from build123d import *

# Parameters (mm, degrees)
F1_DEPTH         = 1
F4_DEPTH         = 0.7
F4_COPIES2_COUNT = 2
F5_W             = 38
F5_H             = 12
F6_DEPTH         = 3
F7_R             = 1.5


# Not quite as in the source:
# - a pattern or mirror of a feature is missing from the dataset's text; its kind, count and spacing are read off the source's solid


with BuildPart() as f1:
    # F0 (on Front) → F1 (new body, symmetric)
    with BuildSketch(Plane.XZ):
        with BuildLine():
            ThreePointArc((25, 31.25), (11.7164027855, 16.2518777716), (0, 0))
            Line((0, 0), (35, 0))
            ThreePointArc((35, 0), (41.1356304071, 16.2798974046), (50, 31.25))
            Line((50, 31.25), (25, 31.25))
        make_face()
        with BuildLine():
            ThreePointArc((75, 62.5), (47.6444357815, 50.6439027497), (25, 31.25))
            Line((25, 31.25), (50, 31.25))
            ThreePointArc((50, 31.25), (60.9207680237, 48.138385581), (75, 62.5))
        make_face()
    extrude(amount=F1_DEPTH, both=True)

    # F2: F1 across plane


with BuildPart() as f1_1:
    add(f1.part)
    add(f1.part.mirror(Plane.XY))

    # F3 (on face) → F4 (cut)
    with BuildSketch(Plane.XZ.offset(1)):
        with BuildLine():
            Line((38.3820565676, 10), (6.9138783475, 10))
            ThreePointArc((6.9138783475, 10), (5.1100506614, 7.5137050995), (3.3446205931, 5))
            Line((3.3446205931, 5), (36.543888556, 5))
            ThreePointArc((36.543888556, 5), (37.4296717705, 7.5122424899), (38.3820565676, 10))
        make_face()
        with BuildLine():
            ThreePointArc((14.7901250767, 20), (12.736458423, 17.5163842045), (10.7230770186, 15))
            Line((10.7230770186, 15), (40.5323833312, 15))
            ThreePointArc((40.5323833312, 15), (41.7401268698, 17.5173495329), (43.0176791325, 20))
            Line((43.0176791325, 20), (14.7901250767, 20))
        make_face()
        with BuildLine():
            ThreePointArc((23.7864537922, 30), (21.4399722373, 27.5198472862), (19.1361704174, 25))
            Line((19.1361704174, 25), (45.8671764928, 25))
            ThreePointArc((45.8671764928, 25), (47.4556813757, 27.5242471055), (49.1187564845, 30))
            Line((49.1187564845, 30), (23.7864537922, 30))
        make_face()
        with BuildLine():
            ThreePointArc((33.5555945556, 40), (30.9391304542, 37.5461308043), (28.4123585311, 35))
            Line((28.4123585311, 35), (52.0223589414, 35))
            ThreePointArc((52.0223589414, 35), (53.5018795741, 37.5221680923), (55.0545103176, 40))
            Line((55.0545103176, 40), (33.5555945556, 40))
        make_face()
        with BuildLine():
            ThreePointArc((46.6278522844, 50), (43.0272085219, 47.5769747675), (39.5350905643, 45))
            Line((39.5350905643, 45), (58.5103303946, 45))
            ThreePointArc((58.5103303946, 45), (60.4389654659, 47.5313247859), (62.4471689161, 50))
            Line((62.4471689161, 50), (46.6278522844, 50))
        make_face()
    f4 = extrude(amount=-F4_DEPTH, mode=Mode.SUBTRACT)

    # F4_copies: F4 across plane
    add(f4.mirror(Plane.ZX), mode=Mode.SUBTRACT)

    # F4_copies1: F4 across plane
    add(f4.mirror(Plane(origin=(0, 0, 0), x_dir=(-1, 0, 0), z_dir=(0, 0, -1))), mode=Mode.SUBTRACT)

    # F4_copies2: F4 ×2 about axis
    f4_copies2_axis = Axis((0, 0, 0), (1, 0, 0))
    for i in range(1, F4_COPIES2_COUNT):
        add(f4.rotate(f4_copies2_axis, i * 360 / F4_COPIES2_COUNT), mode=Mode.SUBTRACT)

    # F5 (on Front) → F6 (join, symmetric)
    with BuildSketch(Plane.XZ):
        with Locations((-13, 0)):
            Rectangle(F5_W, F5_H)
    extrude(amount=F6_DEPTH, both=True)

    # F7
    f7_edges = [f1_1.edges().sort_by_distance(p)[0] for p in [
        (-13, 3, 6),
        (-13, -3, 6),
        (-13, -3, -6),
        (-13, 3, -6),
    ]]
    fillet(f7_edges, radius=F7_R)


solid = f1_1.part
Input: part model. Units: mm. Frame: model coordinates. A direction names the side the tool comes from. Give positions to 0.01 mm unless a question says otherwise; leave off trailing zeros. Order: outer loops, then holes, each group sorted by start corner. A loop starts at its lowest first (then second) coordinate and runs counter-clockwise, first axis right, second up.
Q1. Section B-B on x = 64.5. Output: boundary loops of the cut face in (y, z), and give its area (3 significant figures).
Checked values:
outline: (-1, -59.08) - (1, -59.08) - (1, -52.37) - (-1, -52.37) - close; (-1, 52.37) - (1, 52.37) - (1, 59.08) - (-1, 59.08) - close
area: 26.9 mm2
Q2. Contact query for flat-ended pins moving along their axis: pin 1 Ø0.8 at (x, y) = (45, -1) entering from +Z; pin 2 Ø0.6 at (x, y) = (30, 0.5) entering from -Z; pin 3 Ø0.8 at (x, y) = (35.5, -0.5) entering from +Z. Output: stop coordinate, or through.
Checked values:
pin 1: stops at z = 45
pin 2: stops at z = -36.84
pin 3: stops at z = 42.06
Q3. Section A-A on x = 1.5. Output: boundary loops of the cut face in (y, z).
Checked values:
outline: (-3, -4.5) arc R1.5 ccw to (-1.5, -6) - (1.5, -6) arc R1.5 ccw to (3, -4.5) - (3, 4.5) arc R1.5 ccw to (1.5, 6) - (-1.5, 6) arc R1.5 ccw to (-3, 4.5) - close
Q4. Section D-D on z = -33.5. Output: boundary loops of the cut face in (x, y).
Checked values:
outline: (27.01, -1) - (51.19, -1) - (51.19, 1) - (27.01, 1) - close
Q5. Section C-C on z = 52.5. Output: boundary loops of the cut face in (x, y).
Checked values:
outline: (50.74, -1) - (64.62, -1) - (64.62, 1) - (50.74, 1) - close
Q6. Set-up query: faces 4 (the flat face through (27, 0.3, -18)), 5 (the cylindrical face through (41, 0, 16)), 6 (the flat face through (51, -0.3, -48)). Return all of +Z, -Z, +X, -X, +Y, -Y with unobstructed straight access to the full face (end or side cutting, diameter ignored); none if empty.
Checked values:
face 4: +X, -X, +Y
face 5: +X, +Y, -Y
face 6: +X, -X, -Y
Q7. Draft query along Z for faces 1 (the flat face through (38, 1, 32)), 2 (the flat face through (-13, 0, -6)), 3 (the flat face through (34, -0.3, -28)). Return one class per face: +Z half, -Z half, draft (parallel to the pull), parting line (faces both ways), or undercut.
Checked values:
face 1: draft
face 2: -Z half
face 3: undercut
Q8. Ray query, probe 1 along Z at (x, y) = (-5, -0.3); probe 2 along Y at (x, z) = (33, 31); probe 3 along Y at (x, z) = (32, 6). Return the intervals inside material, ascending.
Checked values:
probe 1: z = -6 to 6
probe 2: y = -1 to 1
probe 3: y = -0.3 to 0.3
